```python
from build123d import *

# Parameters (mm, degrees)
SKETCH1_R           = 2
BOSS_EXTRUDE1_DEPTH = 12
CUT_EXTRUDE1_DEPTH  = 144.178202252
FILLET1_R           = 2


with BuildPart() as part:
    # Sketch1 → Boss-Extrude1 (new body)
    with BuildSketch(Plane(origin=(0, 0, 0), x_dir=(1, 0, 0), z_dir=(0, 1, 0))):
        with BuildLine():
            Line((5.5, 20.76), (128.5, 20.76))
            ThreePointArc((128.5, 20.76), (129.207106781, 20.467106781), (129.5, 19.76))
            Line((129.5, 19.76), (129.5, -3.5))
            ThreePointArc((129.5, -3.5), (129.792893219, -4.207106781), (130.5, -4.5))
            Line((130.5, -4.5), (137.5, -4.5))
            ThreePointArc((137.5, -4.5), (138.207106781, -4.207106781), (138.5, -3.5))
            Line((138.5, -3.5), (138.5, 28.76))
            ThreePointArc((138.5, 28.76), (138.207106781, 29.467106781), (137.5, 29.76))
            Line((137.5, 29.76), (-3.5, 29.76))
            ThreePointArc((-3.5, 29.76), (-4.207106781, 29.467106781), (-4.5, 28.76))
            Line((-4.5, 28.76), (-4.5, 17.76))
            ThreePointArc((-4.5, 17.76), (-4.207106781, 17.052893219), (-3.5, 16.76))
            Line((-3.5, 16.76), (3.5, 16.76))
            ThreePointArc((3.5, 16.76), (4.207106781, 17.052893219), (4.5, 17.76))
            Line((4.5, 17.76), (4.5, 19.76))
            ThreePointArc((4.5, 19.76), (4.792893219, 20.467106781), (5.5, 20.76))
        make_face()
        with Locations(Location((0, 21.76, 0), (0, 0, 270))):
            Circle(SKETCH1_R, mode=Mode.SUBTRACT)
        with Locations(Location((134, 0, 0), (0, 0, 270))):
            Circle(SKETCH1_R, mode=Mode.SUBTRACT)
    extrude(amount=BOSS_EXTRUDE1_DEPTH)

    # Sketch2 → Cut-Extrude1 (cut, through all)
    with BuildSketch(Plane.XY.offset(4.5)):
        Polygon((-4.5, 12), (-4.5, 2), (6.671572875, 2), (16.671572875, 12), align=None)
        Polygon((7.5, 0), (123.5, 0), (113.5, 10), (17.5, 10), align=None)
        Polygon((114.328427125, 12), (124.328427125, 2), (138.5, 2), (138.5, 12), align=None)
    extrude(amount=-CUT_EXTRUDE1_DEPTH, mode=Mode.SUBTRACT)

    # Fillet1
    fillet1_edges = [part.edges().sort_by_distance(p)[0] for p in [
        (16.671572875, 12, -25.26),
        (6.671572875, 2, -25.26),
        (7.5, 0, -25.26),
        (17.5, 10, -25.26),
        (113.5, 10, -25.26),
        (123.5, 0, -25.26),
        (124.328427125, 2, -25.26),
        (114.328427125, 12, -25.26),
    ]]
    fillet(fillet1_edges, radius=FILLET1_R)


solid = part.part
```
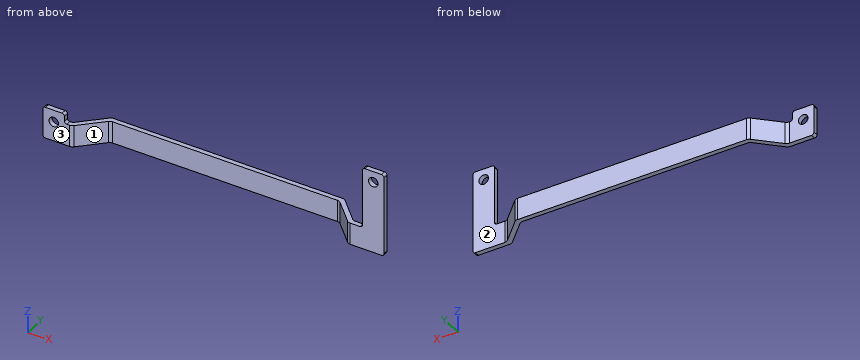
Source: CAD feature listing. Evaluate the final solid. Frame: model axes, mm. Face numbers are marked on the shaded views. A direction names the side the tool comes from. Round coordinates to 2 decimals unless told otherwise and drop trailing zeros. Loops run counter-clockwise (first coordinate to the right, second up) from the corner with the lowest first, then second, coordinate; pieces in that order, holes last. Notation, with made-up numbers: (48.5, 31.25) - (77.5, 31.25) arc R19 ccw to (77.5, 41.25) - close; hole circle Ø1 at (16.5, 7). An arc over 180 degrees is marked (long way). Use CSV: the item, a comma, the result in double quotes.
Q1. Ray query, line 1 along X through (y, z) = (1.05, 0); line 2 along Z through (x, y) = (134, 1.5); line 3 along X through (y, z) = (0.65, -21.76). Return the intervals inside material, ascending.
Reported:
line 1,"129.5 to 132, 136 to 138.5"
line 2,"-29.76 to -2, 2 to 4.5"
line 3,"-4.5 to -2, 2 to 8.15, 122.85 to 138.5"
Q2. Section query D-D, the plane z = -15. Output: boundary loops of the cut face in (x, y).
Reported:
outline,"(129.5, 0) - (138.5, 0) - (138.5, 2) - (129.5, 2) - close"
Q3. Section query A-A, the plane x = 0. Output: boundary loops of the cut face in (y, z), then the cut area to 3 significant figures.
Reported:
outline,"(0, -29.76) - (2, -29.76) - (2, -23.76) - (0, -23.76) - close; (0, -19.76) - (2, -19.76) - (2, -16.76) - (0, -16.76) - close"
area,"18.0 mm^2"
Q4. Reachability of the marked faces 1, 2 and 3 from +Z, -Z, +X, -X, +Y, -Y: full face, straight path, thin tool, end or side. Return the list, or none.
Reported:
face 1,"+Z, -Z, -Y"
face 2,"+Z, -Z, +X, +Y"
face 3,"+Z, -Z, +X, -X, -Y"
Q5. Section query B-B, the plane z = 0. Output: boundary loops of the cut face in (x, y), then the cut area to 3 significant figures.
Reported:
outline,"(129.5, 0) - (132, 0) - (132, 2) - (129.5, 2) - close; (136, 0) - (138.5, 0) - (138.5, 2) - (136, 2) - close"
area,"10.0 mm^2"
Q6. Pin query (flat end, axial travel): pin 1 Ø1.6 at (y, z) = (1, -13) entering from -X; pin 2 Ø0.6 at (x, y) = (1.5, 0.5) entering from +Z; pin 3 Ø14.5 at (x, z) = (133, -9.5) entering from +Y. Return the tip coordinate at first contact, or that it passes through.
Reported:
pin 1,"x = 129.5"
pin 2,"z = -16.76"
pin 3,"y = 2"
Q7. Section query C-C, the plane x = 34. Output: boundary loops of the cut face in (y, z), then the cut area to 3 significant figures.
Reported:
outline,"(10, -29.76) - (12, -29.76) - (12, -20.76) - (10, -20.76) - close"
area,"18.0 mm^2"
